Source: CAD feature listing. Evaluate the final solid. Frame: model axes, mm. Coordinates: 2 decimals unless noted, no trailing zeros. Order: outer loops, then holes, each group sorted by start corner. A loop starts at its lowest first (then second) coordinate and runs counter-clockwise, first axis right, second up.
```python
from build123d import *

# Parameters (mm, degrees)
SKETCH_1_W      = 30
SKETCH_1_H      = 2
EXTRUDE_2_DEPTH = 2


with BuildPart() as part:
    # 草图1 → 凸台-拉伸2 (new body)
    with BuildSketch(Plane.XY):
        Polygon((-8, -36.22154055), (-10, -36.22154055), (-10, -56.22154055), (-8, -56.22154055), (-8, -76.22154055), (-10, -76.22154055), (-10, -96.22154055), (-8, -96.22154055), (-8, -116.22154055), (-10, -116.22154055), (-10, -136.22154055), (-8, -136.22154055), (-8, -156.22154055), (-10, -156.22154055), (-10, -174), (-8, -174), (27, -174), (29, -174), (29, -156.22154055), (27, -156.22154055), (27, -136.22154055), (29, -136.22154055), (29, -116.22154055), (27, -116.22154055), (27, -96.22154055), (29, -96.22154055), (29, -76.22154055), (27, -76.22154055), (27, -56.22154055), (29, -56.22154055), (29, -36.22154055), (27, -36.22154055), (27, -16.22154055), (29, -16.22154055), (29, 3.77845945), (27, 3.77845945), (27, 23.77845945), (29, 23.77845945), (29, 43.77845945), (27, 43.77845945), (27, 49), (27, 59), (-10, 59), (-10, 49), (-8, 49), (-8, 45), (2, 45), (2, 43.34252786), (2, 15.14100393), (2, -15.14100393), (2, -31.22154055), (2, -32.22154055), (-8, -32.22154055), align=None)
        with Locations((9.5, -95.22154055)):
            Rectangle(SKETCH_1_W, SKETCH_1_H, mode=Mode.SUBTRACT)
        with Locations((9.5, -135.22154055)):
            Rectangle(SKETCH_1_W, SKETCH_1_H, mode=Mode.SUBTRACT)
        with Locations((9.5, -55.22154055)):
            Rectangle(SKETCH_1_W, SKETCH_1_H, mode=Mode.SUBTRACT)
    extrude(amount=EXTRUDE_2_DEPTH)


solid = part.part
```
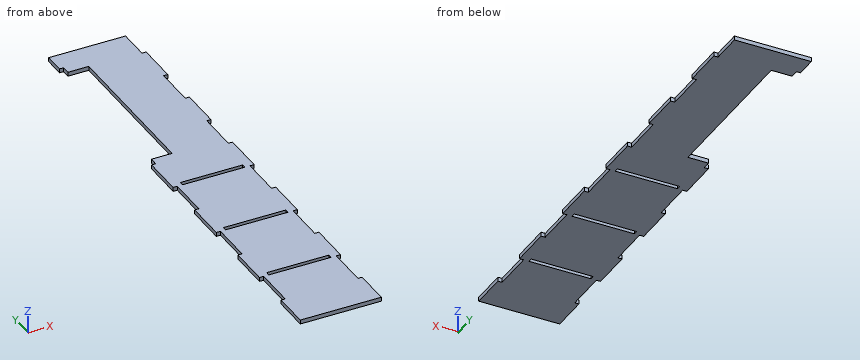
1. Section query D-D on y = -153. Return loops of the section in (x, z).
Findings:
outline: (-8, 0) - (27, 0) - (27, 2) - (-8, 2) - close
2. Pin query (flat end, axial travel): P1, Ø1, axis at y = 48, z = 1.5, coming from the +X side; P2, Ø1, axis at y = -66.5, z = 1, coming from the -X side. Return the tip coordinate at first contact, or that it passes through.
Findings:
P1: stops at x = 27
P2: stops at x = -8
3. Section query B-B on x = 14. Return loops of the section in (y, z).
Findings:
outline: (-174, 0) - (-136.22, 0) - (-136.22, 2) - (-174, 2) - close; (-134.22, 0) - (-96.22, 0) - (-96.22, 2) - (-134.22, 2) - close; (-94.22, 0) - (-56.22, 0) - (-56.22, 2) - (-94.22, 2) - close; (-54.22, 0) - (59, 0) - (59, 2) - (-54.22, 2) - close
4. Section query C-C on z = 0.7. Count the separate pieces of the cut face and the enclosed holes in it, plus the area to 3 significant figures.
Findings:
separate pieces: 1
enclosed holes: 3
area: 7,610 mm2
5. Ray query, line 1 (Y direction, x = 0, z = 1.45); line 2 (Y direction, x = 17, z = 0.3); line 3 (X direction, y = -1, z = 0.75). Return the intervals inside material, ascending.
Findings:
line 1: y = -174 to -136.22, -134.22 to -96.22, -94.22 to -56.22, -54.22 to -32.22, 45 to 59
line 2: y = -174 to -136.22, -134.22 to -96.22, -94.22 to -56.22, -54.22 to 59
line 3: x = 2 to 29
6. Section query A-A on x = -1. Return loops of the section in (y, z).
Findings:
outline: (-174, 0) - (-136.22, 0) - (-136.22, 2) - (-174, 2) - close; (-134.22, 0) - (-96.22, 0) - (-96.22, 2) - (-134.22, 2) - close; (-94.22, 0) - (-56.22, 0) - (-56.22, 2) - (-94.22, 2) - close; (-54.22, 0) - (-32.22, 0) - (-32.22, 2) - (-54.22, 2) - close; (45, 0) - (59, 0) - (59, 2) - (45, 2) - close
